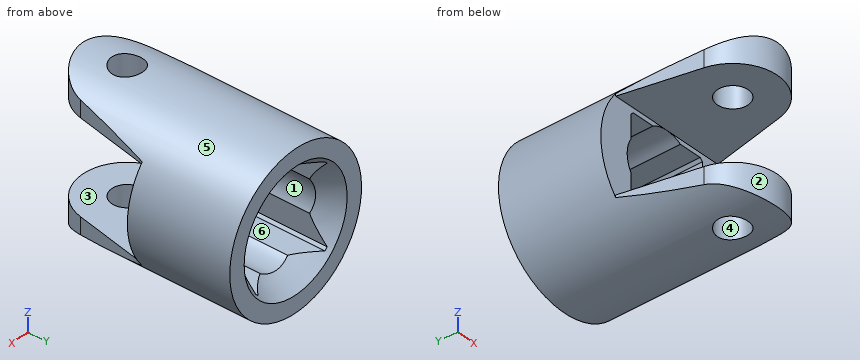
from build123d import *

# Parameters (mm, degrees)
SKETCH1_R           = 12
BOSS_EXTRUDE1_DEPTH = 33.53
CUT_EXTRUDE1_DEPTH  = 19.6
CHAMFER1_SIZE       = 0.4
SKETCH3_R           = 9.375
CUT_EXTRUDE2_DEPTH  = 3.4
CUT_EXTRUDE2_DRAFT  = -35
SKETCH4_W           = 24
SKETCH4_H           = 14.42225279
CUT_EXTRUDE3_DEPTH  = 17.4
SKETCH5_R           = 2.415
CUT_EXTRUDE4_DEPTH  = 33.7


with BuildPart() as part:
    # Sketch1 → Boss-Extrude1 (new body)
    with BuildSketch(Plane(origin=(0, 0, 0), x_dir=(1, 0, 0), z_dir=(0, 1, 0))):
        with Locations(Location((0, 0, 0), (0, 0, 270))):
            Circle(SKETCH1_R)
    extrude(amount=BOSS_EXTRUDE1_DEPTH)

    # Sketch2 → Cut-Extrude1 (cut)
    with BuildSketch(Plane(origin=(0, 33.53, 0), x_dir=(1, 0, 0), z_dir=(0, 1, 0))):
        with BuildLine():
            Line((-6.5, 6.5), (-2.5, 6.5))
            ThreePointArc((-2.5, 6.5), (0, 7.211126395), (2.5, 6.5))
            Line((2.5, 6.5), (6.5, 6.5))
            Line((6.5, 6.5), (6.5, 2.5))
            ThreePointArc((6.5, 2.5), (7.211126395, 0), (6.5, -2.5))
            Line((6.5, -2.5), (6.5, -6.5))
            Line((6.5, -6.5), (2.5, -6.5))
            ThreePointArc((2.5, -6.5), (0, -7.211126395), (-2.5, -6.5))
            Line((-2.5, -6.5), (-6.5, -6.5))
            Line((-6.5, -6.5), (-6.5, -2.5))
            ThreePointArc((-6.5, -2.5), (-7.211126395, 0), (-6.5, 2.5))
            Line((-6.5, 2.5), (-6.5, 6.5))
        make_face()
    extrude(amount=-CUT_EXTRUDE1_DEPTH, mode=Mode.SUBTRACT)

    # Chamfer1
    chamfer1_edges = [part.edges().sort_by_distance(p)[0] for p in [
        (-6.5, 23.73, -6.5),
        (6.5, 23.73, -6.5),
        (6.5, 23.73, 6.5),
        (-6.5, 23.73, 6.5),
    ]]
    chamfer(chamfer1_edges, length=CHAMFER1_SIZE)


with BuildPart() as cut_extrude2_tool:
    # Sketch3 → Cut-Extrude2 (with draft: the straight prism first)
    with BuildSketch(Plane(origin=(0, 33.53, 0), x_dir=(1, 0, 0), z_dir=(0, 1, 0))):
        Circle(SKETCH3_R)
    extrude(amount=-CUT_EXTRUDE2_DEPTH)
    # Cut-Extrude2: the draft: its side faces are tilted about the plane it starts from
    cut_extrude2_sides = [cut_extrude2_tool.faces().sort_by_distance(p)[0] for p in [
        (-9.375, 31.83, 0),
    ]]
    draft(cut_extrude2_sides, Plane(origin=(0, 33.53, 0), x_dir=(1, 0, 0), z_dir=(0, 1, 0)), CUT_EXTRUDE2_DRAFT)


with BuildPart() as part_1:
    add(part.part)

    # Cut-Extrude2: cut by cut_extrude2_tool
    add(cut_extrude2_tool.part, mode=Mode.SUBTRACT)

    # Sketch4 → Cut-Extrude3 (cut)
    with BuildSketch(Plane.XZ):
        Rectangle(SKETCH4_W, SKETCH4_H)
    extrude(amount=-CUT_EXTRUDE3_DEPTH, mode=Mode.SUBTRACT)

    # Sketch5 → Cut-Extrude4 (cut, symmetric)
    with BuildSketch(Plane.XY):
        with Locations(Location((0, 7, 0), (0, 0, 90))):
            Circle(SKETCH5_R)
        with BuildLine():
            ThreePointArc((-6.854820161, 5.581747356), (0, 0), (6.854820161, 5.581747356))
            Line((6.854820161, 5.581747356), (9.3, 17.4))
            Line((9.3, 17.4), (12, 17.4))
            Line((12, 17.4), (12, -3.192277431))
            Line((12, -3.192277431), (-12, -3.192277431))
            Line((-12, -3.192277431), (-12, 17.4))
            Line((-12, 17.4), (-9.3, 17.4))
            Line((-9.3, 17.4), (-6.854820161, 5.581747356))
        make_face()
    extrude(amount=CUT_EXTRUDE4_DEPTH, both=True, mode=Mode.SUBTRACT)


solid = part_1.part
Could you check a few things on this model? Use its own coordinates, in mm. Face numbers are marked on the shaded views. A direction names the side the tool comes from. Give positions to 0.01 mm unless a question says otherwise; leave off trailing zeros. Loops run counter-clockwise (first coordinate to the right, second up) from the corner with the lowest first, then second, coordinate; pieces in that order, holes last. Notation, with made-up numbers: (73.25, -5.75) -> (100.25, -5.75) arc R12 cw to (100.25, 16.25) -> close; hole circle Ø11 at (-24, 18). An arc over 180 degrees is marked (long way). Return JSON: item names as keys, results as strings.
Item 1: If we section it at C-C on y = 7: List the corners of the cut face in (x, z) for me (3 decimals), plus the area to 3 significant figures.
Geometry results:
{"outline": "(-7.148, -9.639) arc R12 ccw to (-2.415, -11.754) -> (-2.415, -7.211) -> (-7.148, -7.211) -> close; (-7.148, 7.211) -> (-2.415, 7.211) -> (-2.415, 11.754) arc R12 ccw to (-7.148, 9.639) -> close; (2.415, -11.754) arc R12 ccw to (7.148, -9.639) -> (7.148, -7.211) -> (2.415, -7.211) -> close; (2.415, 7.211) -> (7.148, 7.211) -> (7.148, 9.639) arc R12 ccw to (2.415, 11.754) -> close", "area": "69.9 mm²"}
Item 2: Which directions (+Z, -Z, +X, -X, +Y, -Y) give clear straight access to the entire face, cutting with the end or side of a thin tool? Please do the marked faces 1, 2 and 3.
Geometry results:
{"face 1": "+Y, -Y", "face 2": "+Z, -Z, -Y", "face 3": "+X, -X, -Y"}
Item 3: If we section it at A-A on z = 0: List the corners of the cut face in (x, y) for me (3 decimals), plus the area to 3 significant figures.
Geometry results:
{"outline": "(-12, 17.4) -> (-7.211, 17.4) -> (-7.211, 30.44) -> (-9.375, 33.53) -> (-12, 33.53) -> close; (7.211, 17.4) -> (12, 17.4) -> (12, 33.53) -> (9.375, 33.53) -> (7.211, 30.44) -> close", "area": "148 mm²"}
Item 4: I need wall thicknesses on L1, parallel to Y at x = 0, z = 9.55 (3 decimals); L2, parallel to X at y = 7, z = 9.15 (3 decimals); L3, parallel to Z at x = 6, y = 18. Which ranges of each line are inside material? Lowest first, please. Write a range as from..to.
Geometry results:
{"L1": "y = 0..4.585, 9.415..33.53", "L2": "x = -7.148..-2.415, 2.415..7.148", "L3": "z = -10.39..-6.5, 6.5..10.39"}
Item 5: We'd pull the mould along Z, two halves only. Please class the marked faces 4, 5 and 6: +Z half, -Z half, draft (parallel to the pull), parting line (faces both ways), or undercut.
Geometry results:
{"face 4": "draft", "face 5": "parting line", "face 6": "undercut"}
Item 6: If we section it at D-D on y = 15.5: List the corners of the cut face in (x, z) for me.
Geometry results:
{"outline": "(-8.91, -8.04) arc R12 ccw to (8.91, -8.04) -> (8.91, -7.21) -> (-8.91, -7.21) -> close; (-8.91, 7.21) -> (8.91, 7.21) -> (8.91, 8.04) arc R12 ccw to (-8.91, 8.04) -> close"}
Item 7: If we section it at B-B on y = 21.5: List the corners of the cut face in (x, z) for me, plus the area to 3 significant figures.
Geometry results:
{"outline": "circle Ø24 at (0, 0); hole (-6.5, -6.1) -> (-6.1, -6.5) -> (-2.5, -6.5) arc R4.75 ccw to (2.5, -6.5) -> (6.1, -6.5) -> (6.5, -6.1) -> (6.5, -2.5) arc R4.75 ccw to (6.5, 2.5) -> (6.5, 6.1) -> (6.1, 6.5) -> (2.5, 6.5) arc R4.75 ccw to (-2.5, 6.5) -> (-6.1, 6.5) -> (-6.5, 6.1) -> (-6.5, 2.5) arc R4.75 ccw to (-6.5, -2.5) -> close", "area": "274 mm²"}
Item 8: I'm going to push flat-ended pins straight in: pin 1 (4 mm diameter, centred on x = -3.5, y = 22, fed in from +Z); pin 2 (6 mm diameter, centred on x = 6, z = -1, fed in from -Y); pin 3 (6 mm diameter, centred on x = 5.5, y = 20, fed in from +Z); pin 4 (6.5 mm diameter, centred on x = 0, y = 7, fed in from -Z). Where does each tip first touch, or does it pass through?
Geometry results:
{"pin 1": "stops at z = 11.91", "pin 2": "stops at y = 17.4", "pin 3": "stops at z = 11.74", "pin 4": "stops at z = -12"}
